```python
from build123d import *

# Parameters (mm, degrees)
BOSS_EXTRUDE1_DEPTH = 3
BOSS_EXTRUDE2_DEPTH = 4.25
CUT_EXTRUDE1_DEPTH  = 1.2
CUT_EXTRUDE2_START  = -1.2
CUT_EXTRUDE2_DEPTH  = 1.2
BOSS_EXTRUDE3_DEPTH = 2
BOSS_EXTRUDE4_DEPTH = 2
FILLET2_R           = 4.5
FILLET3_START       = -18
FILLET3_DEPTH       = 19
FILLET3_START_2     = -16.6
FILLET3_2_DEPTH     = 2
FILLET3_START_3     = -2
FILLET3_3_DEPTH     = 2
SKETCH7_W           = 5
SKETCH7_H           = 1.1
BOSS_EXTRUDE5_DEPTH = 0.7
FILLET4_R           = 0.5


with BuildPart() as part:
    # Sketch1 → Boss-Extrude1 (new body)
    with BuildSketch(Plane(origin=(0, 0, 0), x_dir=(1, 0, 0), z_dir=(0, 1, 0))):
        with BuildLine():
            Line((0, 0), (17, 0))
            ThreePointArc((17, 0), (25.3, 8.3), (17, 16.6))
            Line((17, 16.6), (0, 16.6))
            Line((0, 16.6), (0, 14.6))
            Line((0, 14.6), (6, 14.6))
            Line((6, 14.6), (6, 2))
            Line((6, 2), (0, 2))
            Line((0, 2), (0, 0))
        make_face()
    extrude(amount=BOSS_EXTRUDE1_DEPTH)

    # Sketch2 → Boss-Extrude2 (add)
    with BuildSketch(Plane(origin=(0, 3, 0), x_dir=(1, 0, 0), z_dir=(0, 1, 0))):
        with BuildLine():
            Line((6, 2), (0, 2))
            Line((0, 2), (0, 0))
            Line((0, 0), (17, 0))
            ThreePointArc((17, 0), (25.3, 8.3), (17, 16.6))
            Line((17, 16.6), (0, 16.6))
            Line((0, 16.6), (0, 14.6))
            Line((0, 14.6), (6, 14.6))
            Line((6, 14.6), (17, 14.6))
            ThreePointArc((17, 14.6), (23.3, 8.3), (17, 2))
            Line((17, 2), (6, 2))
        make_face()
    extrude(amount=BOSS_EXTRUDE2_DEPTH)

    # Sketch3 → Cut-Extrude1 (cut)
    with BuildSketch(Plane.XY.offset(-14.6)):
        with BuildLine():
            ThreePointArc((0.762563133, 6.487436867), (0.762563133, 4.012563133), (3.237436867, 4.012563133))
            Line((3.237436867, 4.012563133), (0.762563133, 6.487436867))
        make_face()
        with BuildLine():
            Line((0.762563133, 6.487436867), (3.237436867, 4.012563133))
            ThreePointArc((3.237436867, 4.012563133), (3.616789182, 4.580303993), (3.75, 5.25))
            ThreePointArc((3.75, 5.25), (2.669696007, 6.866789182), (0.762563133, 6.487436867))
        make_face()
    extrude(amount=-CUT_EXTRUDE1_DEPTH, mode=Mode.SUBTRACT)

    # Sketch4 → Cut-Extrude2 (cut)
    with BuildSketch(Plane(origin=(0, 0, -2), x_dir=(-1, 0, 0), z_dir=(0, 0, -1)).offset(CUT_EXTRUDE2_START)):
        with BuildLine():
            ThreePointArc((-0.25, 5.25), (-0.383210818, 5.919696007), (-0.762563133, 6.487436867))
            Line((-0.762563133, 6.487436867), (-3.237436867, 4.012563133))
            ThreePointArc((-3.237436867, 4.012563133), (-1.330303993, 3.633210818), (-0.25, 5.25))
        make_face()
        with BuildLine():
            Line((-3.237436867, 4.012563133), (-0.762563133, 6.487436867))
            ThreePointArc((-0.762563133, 6.487436867), (-3.237436867, 6.487436867), (-3.237436867, 4.012563133))
        make_face()
    extrude(amount=CUT_EXTRUDE2_DEPTH, mode=Mode.SUBTRACT)

    # Sketch5 → Boss-Extrude3 (add)
    with BuildSketch(Plane.XY):
        Polygon((5, 7.25), (5, 9.25), (-2, 9.25), (-2, 0), (0, 0), (0, 7.25), align=None)
    extrude(amount=-BOSS_EXTRUDE3_DEPTH)

    # Sketch6 → Boss-Extrude4 (add)
    with BuildSketch(Plane(origin=(0, 0, -16.6), x_dir=(-1, 0, 0), z_dir=(0, 0, -1))):
        Polygon((-5, 7.25), (-5, 9.25), (2, 9.25), (2, 0), (0, 0), (0, 7.25), align=None)
    extrude(amount=-BOSS_EXTRUDE4_DEPTH)

    # Fillet2
    fillet2_edges = [part.edges().sort_by_distance(p)[0] for p in [
        (-2, 0, -1),
        (-2, 9.25, -1),
        (-2, 9.25, -15.6),
        (-2, 0, -15.6),
    ]]
    fillet(fillet2_edges, radius=FILLET2_R)

    # Fillet3: read off the stored shape, not the designer's step
    # Fillet3 outline → Fillet3 (cut)
    with BuildSketch(Plane.XY.offset(FILLET3_START)):
        with BuildLine():
            Line((5, 9.25), (4, 9.25))
            ThreePointArc((4, 9.25), (4.707106781, 8.957106781), (5, 8.25))
            Line((5, 8.25), (5, 9.25))
        make_face()
    extrude(amount=FILLET3_DEPTH, mode=Mode.SUBTRACT)

    # Fillet3 2 outline → Fillet3 2 (add)
    with BuildSketch(Plane.XY.offset(FILLET3_START_2)):
        with BuildLine():
            ThreePointArc((6, 7.25), (5.292893219, 7.542893219), (5, 8.25))
            Line((5, 8.25), (5, 7.25))
            Line((5, 7.25), (6, 7.25))
        make_face()
    extrude(amount=FILLET3_2_DEPTH)

    # Fillet3 3 outline → Fillet3 3 (add)
    with BuildSketch(Plane.XY.offset(FILLET3_START_3)):
        with BuildLine():
            ThreePointArc((6, 7.25), (5.292893219, 7.542893219), (5, 8.25))
            Line((5, 8.25), (5, 7.25))
            Line((5, 7.25), (6, 7.25))
        make_face()
    extrude(amount=FILLET3_3_DEPTH)

    # Sketch7 → Boss-Extrude5 (add)
    with BuildSketch(Plane(origin=(23.5, 0, 0), x_dir=(0, 0, -1), z_dir=(1, 0, 0))):
        with Locations((8.3, 5.125)):
            Rectangle(SKETCH7_W, SKETCH7_H)
    extrude(amount=-BOSS_EXTRUDE5_DEPTH)

    # Fillet4
    fillet4_edges = [part.edges().sort_by_distance(p)[0] for p in [
        (22.8, 4.575, -8.3),
        (22.8, 5.675, -8.3),
    ]]
    fillet(fillet4_edges, radius=FILLET4_R - 0.0001)  # a hair under: the kernel refuses the full size


solid = part.part
```
The listing builds one solid part. Answer for the finished solid, in the listing's coordinates (mm). A direction names the side the tool comes from. Coordinates: 2 decimals unless noted, no trailing zeros. Write each loop counter-clockwise with the first axis right and the second up, starting at its lowest first coordinate (ties: lowest second). Pieces come first, ordered by that corner, then holes. Notation, with made-up numbers: (49, 50) - (97, 50) arc R25 ccw to (97, 81) - close; hole circle Ø5 at (39.5, 41.5). An arc over 180 degrees is marked (long way). Return JSON: item names as keys, results as strings. Group by question number.
1. A cutting plane is placed at D-D, the plane z = -5.25. Determine the outline of the cut face in (x, y).
2. A cutting plane is placed at B-B, the plane x = 18.25. Determine the outline of the cut face in (y, z).
3. A cutting plane is placed at C-C, the plane y = 1.75. Determine the outline of the cut face in (x, z).
4. Straight lines are drawn through the part: L1, parallel to Z at x = 2, y = 6.75; L2, parallel to Z at x = 17.25, y = 7; L3, parallel to X at y = 5.75, z = -8.5. For each, find the intervals that lie inside material, in ascending order.
5. Which of the six approach directions +Z, -Z, +X, -X, +Y, -Y give full straight-line access (tool end or side, diameter ignored) to faces 1 (the flat face through (2, 5, -0.8)), 2 (the flat face through (19.2, 7.25, -14.5)), 3 (the flat face through (7, 5, -2))?
6. Determine the mould class of faces 4 (the cylindrical face through (23.3, 6, -8.4)), 5 (the flat face through (3, 9.25, -16)), 6 (the flat face through (7, 4, -16.6)), 7 (the flat face through (7, 4, 0)) for opening direction Z: released by +Z, released by -Z, zero draft, split by the parting line, or undercut.
7. A cutting plane is placed at A-A, the plane x = 2. Determine the outline of the cut face in (y, z).
8. Given pin 1 (0.9 mm diameter, centred on y = 1.5, z = -7.5, fed in from -X); pin 2 (1 mm diameter, centred on x = 13, z = -10, fed in from -Y); pin 3 (8.5 mm diameter, centred on x = 15, z = -4.5, fed in from +Y); pin 4 (4 mm diameter, centred on y = 6, z = -7.5, fed in from -X), each flat-ended and moving along its own axis, determine where each tip first touches the part or whether it passes through.
Ans:
{
 "1": {"outline": "(6, 0) - (24.72, 0) - (24.72, 7.25) - (22.51, 7.25) - (22.51, 3) - (6, 3) - close"},
 "2": {"outline": "(0, -16.51) - (7.25, -16.51) - (7.25, -14.47) - (3, -14.47) - (3, -2.13) - (7.25, -2.13) - (7.25, -0.09) - (0, -0.09) - close"},
 "3": {"outline": "(-1.06, -16.6) - (17, -16.6) arc R8.3 ccw to (17, 0) - (-1.06, 0) - (-1.06, -2) - (6, -2) - (6, -14.6) - (-1.06, -14.6) - close"},
 "4": {"L1": "-16.6 to -15.8, -0.8 to 0", "L2": "-16.6 to -14.6, -2 to 0", "L3": "23.3 to 25.3"},
 "5": {"face 1": "none", "face 2": "+Z, -Z, +X, +Y", "face 3": "-X, +Y"},
 "6": {"face 4": "undercut", "face 5": "zero draft", "face 6": "released by -Z", "face 7": "released by +Z"},
 "7": {"outline": "(0.03, -16.6) - (9.22, -16.6) - (9.22, -14.6) - (7, -14.6) - (7, -15.8) - (3.5, -15.8) - (3.5, -14.6) - (0.03, -14.6) - close; (0.03, -2) - (3.5, -2) - (3.5, -0.8) - (7, -0.8) - (7, -2) - (9.22, -2) - (9.22, 0) - (0.03, 0) - close"},
 "8": {"pin 1": "x = 6", "pin 2": "y = 0", "pin 3": "y = 7.25", "pin 4": "x = 22.64"}
}
